Read the model definition and answer for the solid it produces. Units are mm, in the model's axes. A direction names the side the tool comes from. Coordinates: 2 decimals unless noted, no trailing zeros. Put each result on its own line as item: value.
from build123d import *

# Parameters (mm, degrees)
DODANIE_WYCI_GNI_CIE1_DEPTH     = 20
ZAOKR_GLENIE1_R                 = 2
WYTNIJ_WYCI_GNI_CIE1_DEPTH      = 97.32487505
WYTNIJ_WYCI_GNI_CIE1_DEPTH_BACK = 97.32487505
SZKIC4_W                        = 33
SZKIC4_H                        = 47


with BuildPart() as part:
    # Szkic1 → Dodanie-wyciągnięcie1 (new body)
    with BuildSketch(Plane.XY):
        with BuildLine():
            Line((-17.5, -49.947466261), (17.5, -49.947466261))
            ThreePointArc((17.5, -49.947466261), (38.871825844, -25.07740374), (59.999977002, 0))
            ThreePointArc((59.999977002, 0), (55.026266869, 55.026269155), (0, 50.052533739))
            ThreePointArc((0, 50.052533739), (-55.026266869, 55.026269155), (-59.999977002, 0))
            ThreePointArc((-59.999977002, 0), (-38.871825844, -25.07740374), (-17.5, -49.947466261))
        make_face()
    extrude(amount=-DODANIE_WYCI_GNI_CIE1_DEPTH)

    # Zaokrąglenie1
    zaokr_glenie1_edges = [part.edges().sort_by_distance(p)[0] for p in [
        (55.026266869, 55.026269155, -20),
        (38.871825844, -25.07740374, -20),
        (-38.871825844, -25.07740374, -20),
        (38.871825844, -25.07740374, 0),
        (55.026266869, 55.026269155, 0),
        (-55.026266869, 55.026269155, 0),
        (-38.871825844, -25.07740374, 0),
        (-55.026266869, 55.026269155, -20),
        (-17.5, -49.947466261, -10),
        (17.5, -49.947466261, -10),
        (0, 50.052533739, -10),
    ]]
    fillet(zaokr_glenie1_edges, radius=ZAOKR_GLENIE1_R)

    # Szkic4 → Wytnij-wyciągnięcie1 (cut, two sides: drawn at the far end of the back side and taken through both)
    with BuildSketch(Plane.XY.offset(-WYTNIJ_WYCI_GNI_CIE1_DEPTH_BACK)):
        Rectangle(SZKIC4_W, SZKIC4_H)
    extrude(amount=WYTNIJ_WYCI_GNI_CIE1_DEPTH + WYTNIJ_WYCI_GNI_CIE1_DEPTH_BACK, mode=Mode.SUBTRACT)


solid = part.part
1) Which of the six approach directions +Z, -Z, +X, -X, +Y, -Y give full straight-line access (tool end or side, diameter ignored) to faces 5 (the flat face through (0, -49.947, -10)), 6 (the flat face through (16.5, 0, -10))?
Answer list:
face 5: +Z, -Z, +X, -X, -Y
face 6: +Z, -Z
2) Determine the mould class of faces 1 (the flat face through (-1, 32, 0)), 2 (the flat face through (0, -23.5, -10)), 3 (the flat face through (0, 23.5, -10)), 4 (the cylindrical face through (-39.461, -24.385, -9.888)) for opening direction Y: released by +Y, released by -Y, zero draft, split by the parting line, or undercut.
Answer list:
face 1: zero draft
face 2: undercut
face 3: undercut
face 4: released by -Y
3) Given pin 1 Ø1.5 at (x, z) = (44, -16.5) entering from -Y; pin 2 Ø4 at (y, z) = (52, -2) entering from +X; pin 3 Ø10 at (y, z) = (0.5, -14.5) entering from +X, each flat-ended and moving along its own axis, determine where each tip first touches the part or whether it passes through.
Answer list:
pin 1: stops at y = -19.92
pin 2: stops at x = 60.04
pin 3: stops at x = 63.84
4) Straight lines are drawn through the part: line 1 (X direction, y = 17.5, z = -14); line 2 (X direction, y = 20.5, z = -2.25); line 3 (Y direction, x = -9, z = -11). For each, find the intervals that lie inside material, in ascending order. Write a range as [from, to].
Answer list:
line 1: x = [-68.34, -16.5], [16.5, 68.34]
line 2: x = [-68.8, -16.5], [16.5, 68.8]
line 3: y = [-49.95, -23.5], [23.5, 57.97]
